The model under review builds one solid part; all positions refer to its coordinate system, in mm. A direction names the side the tool comes from. Give positions to 0.01 mm unless a question says otherwise; leave off trailing zeros. Write each loop counter-clockwise with the first axis right and the second up, starting at its lowest first coordinate (ties: lowest second). Pieces come first, ordered by that corner, then holes. Notation, with made-up numbers: M 6,3 L 62,3 A16 ccw 62,29 Z; hole C -3,-3 d1. An arc over 180 degrees is marked long. Write item = value, one per line. Start each with the question number.
```python
from build123d import *

# Parameters (mm, degrees)
SKETCH1_R           = 19.05
SKETCH1_R_2         = 5
SKETCH1_R_3         = 2.1
SKETCH1_W           = 3.175
SKETCH1_H           = 3.175
BOSS_EXTRUDE1_DEPTH = 4
BOSS_EXTRUDE2_START = 4
SKETCH1_3_R         = 5
SKETCH1_3_W         = 3.175
SKETCH1_3_H         = 3.175
BOSS_EXTRUDE2_DEPTH = 4.85
FILLET1_R           = 4
FILLET2_R           = 1
FILLET3_R           = 2


with BuildPart() as part:
    # Sketch1 → Boss-Extrude1 (new body)
    # profile 1 of 2: a face of its own
    with BuildSketch(Plane.XY):
        Circle(SKETCH1_R)
        Circle(SKETCH1_R_2, mode=Mode.SUBTRACT)
        with Locations((12.7, 0)):
            Circle(SKETCH1_R_3, mode=Mode.SUBTRACT)
        with Locations((0, -12.7)):
            Circle(SKETCH1_R_3, mode=Mode.SUBTRACT)
        with Locations((-12.7, 0)):
            Circle(SKETCH1_R_3, mode=Mode.SUBTRACT)
        with Locations((0, 12.7)):
            Circle(SKETCH1_R_3, mode=Mode.SUBTRACT)
    # profile 2 of 2: a face of its own
    with BuildSketch(Plane.XY):
        Circle(SKETCH1_R_2)
        Rectangle(SKETCH1_W, SKETCH1_H, mode=Mode.SUBTRACT)
    extrude(amount=BOSS_EXTRUDE1_DEPTH)

    # Sketch1<3> → Boss-Extrude2 (add)
    with BuildSketch(Plane.XY.offset(BOSS_EXTRUDE2_START)):
        Circle(SKETCH1_3_R)
        Rectangle(SKETCH1_3_W, SKETCH1_3_H, mode=Mode.SUBTRACT)
    extrude(amount=BOSS_EXTRUDE2_DEPTH)

    # Fillet1
    fillet1_edges = [part.edges().sort_by_distance(p)[0] for p in [
        (-5, 0, 4),
    ]]
    fillet(fillet1_edges, radius=FILLET1_R)

    # Fillet2
    fillet2_edges = [part.edges().sort_by_distance(p)[0] for p in [
        (-5, 0, 8.85),
    ]]
    fillet(fillet2_edges, radius=FILLET2_R)

    # Fillet3
    fillet3_edges = [part.edges().sort_by_distance(p)[0] for p in [
        (-19.05, 0, 0),
        (-19.05, 0, 4),
    ]]
    fillet(fillet3_edges, radius=FILLET3_R - 0.0001)  # a hair under: the kernel refuses the full size


solid = part.part
```
Item 1: We need section C-C, the plane z = 5. Write out the cut boundary in (x, y).
Item 2: We need section B-B, the plane z = 7.25. Write out the cut boundary in (x, y), and give its area (3 significant figures).
Item 3: To check wall thickness, follow probe 1 along X at (y, z) = (-1, 3.5); probe 2 along Y at (x, z) = (0, 1.1); probe 3 along X at (y, z) = (-1, 1.25). State the ranges of each line that lie inside material, in increasing order. Write a range as [from, to].
Item 4: For faces 1 (the flat face through (1.588, 0, 4)), 2 (the flat face through (0, -4, 0)), 3 (the flat face through (7, -7, 4)), list the 3-axis set-ups (+Z, -Z, +X, -X, +Y, -Y) from which the entire face can be reached by the end or side of a thin tool; tool diameter is ignored.
Item 5: Clearance check with flat-ended pins moving along their axes: P1, Ø2.5, axis at x = -0.5, z = 5, coming from the -Y side; P2, Ø5, axis at y = -10.5, z = 1.5, coming from the +X side; P3, Ø5.5, axis at x = 12.7, y = 0, coming from the +Z side; P4, Ø2.5, axis at x = -12.7, y = 0, coming from the -Z side. State where each tip first meets the part, or that it passes through.
Item 6: We need section A-A, the plane x = 0. Give the number of separate pieces and of enclosed holes in the cut face, and give its area (3 significant figures).
Item 7: The part is to be moulded in two halves that separate along Y. For faces 4 (the flat face through (0, 2, 8.85)), 5 (the cylindrical face through (14.703, 0.631, 1.972)), say which applies: released by +Y, released by -Y, zero draft, split by the parting line, or undercut.
Worked out:
q1.outline = C 0,0 d12.71; hole M -1.59,-1.59 L 1.59,-1.59 L 1.59,1.59 L -1.59,1.59 Z
q2.outline = C 0,0 d10.14; hole M -1.59,-1.59 L 1.59,-1.59 L 1.59,1.59 L -1.59,1.59 Z
q2.area = 70.7 mm²
q3.probe_1 = [-18.35, -14.55], [-10.85, -1.59], [1.59, 10.85], [14.55, 18.35]
q3.probe_2 = [-18.84, -14.8], [-10.6, -1.59], [1.59, 10.6], [14.8, 18.84]
q3.probe_3 = [-18.88, -14.55], [-10.85, -1.59], [1.59, 10.85], [14.55, 18.88]
q4.face_1 = +Z, -Z
q4.face_2 = -Z, +X, -X, +Y, -Y
q4.face_3 = +Z
q5.P1 = -18.01
q5.P2 = 17.27
q5.P3 = 4
q5.P4 = through
q6.separate_pieces = 4
q6.enclosed_holes = 0
q6.area = 142 mm²
q7.face_4 = zero draft
q7.face_5 = undercut
